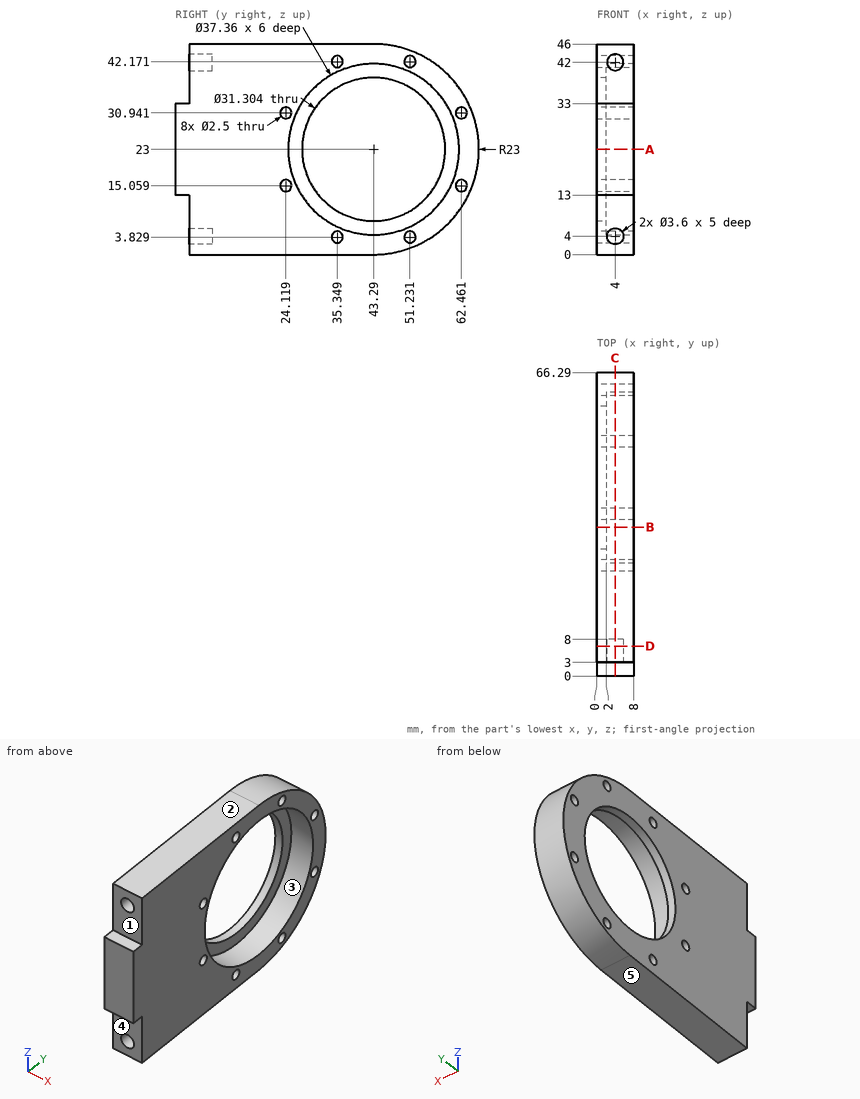
Verification items for this drawing (mm, ordinates from the low corner). A direction names the side the tool comes from. Give positions to 0.01 mm unless a question says otherwise; leave off trailing zeros. Write each loop counter-clockwise with the first axis right and the second up, starting at its lowest first coordinate (ties: lowest second). Pieces come first, ordered by that corner, then holes. Notation, with made-up numbers: M -37,62.25 L -9,62.25 A10 ccw -9,69.25 Z; hole C -33.5,-9.5 d6. An arc over 180 degrees is marked long. Use one line per item in the form item = value.
(1) Draft check along Z on the marked faces 3, 4 and 5. Enter one of: pulls with the +Z half, pulls with the -Z half, needs draft (parallel to the pull), parting line crosses it, or undercut.
Answer block:
face_3 = undercut
face_4 = needs draft
face_5 = pulls with the -Z half
(2) Tool access check on the marked faces 1 and 2. Record the directions out of +Z, -Z, +X, -X, +Y, -Y that give a thin tool (end or side, any length) a straight path to the whole face; none if there is none.
Answer block:
face_1 = +Z, +X, -X, -Y
face_2 = +Z, +X, -X, +Y, -Y
(3) Section check B-B on y = 32.5. Record the boundary of the cut face in (x, z).
Answer block:
outline = M 0,0 L 8,0 L 8,7.75 L 2,7.75 L 2,11.66 L 0,11.66 Z; M 0,34.34 L 2,34.34 L 2,38.25 L 8,38.25 L 8,46 L 0,46 Z
(4) Material ranges on line 1 along X through (y, z) = (6, 4); line 2 along Y through (x, z) = (1.25, 16) (1 decimal); line 3 along Y through (x, z) = (3.75, 30.5), recorded low to high.
Answer block:
line_1 = 0 to 2.2, 5.8 to 8
line_2 = 0 to 23.3, 24.9 to 29.3, 57.3 to 61.6, 63.3 to 65.2
line_3 = 0 to 22.95, 25.29 to 26.18, 60.4 to 61.29, 63.63 to 65.03
(5) Depth check by flat-ended pin: P1, Ø0.9, axis at x = 5, y = 2, coming from the -Z side; P2, Ø19, axis at y = 43.29, z = 23, coming from the -X side; P3, Ø1.8, axis at x = 3.5, z = 4.5, coming from the -Y side; P4, Ø3.5, axis at x = 4, y = 1, coming from the +Z side. Enter the tip coordinate at first touch or a pass-through.
Answer block:
P1 = 13
P2 = through
P3 = 8
P4 = 33
(6) Section check C-C on x = 4. State how many separate pieces and enclosed holes the cut face has, plus the area to 3 significant figures.
Answer block:
separate_pieces = 1
enclosed_holes = 9
area = 1,570 mm2
(7) Section check A-A on z = 23. Record the boundary of the cut face in (x, y).
Answer block:
outline = M 0,0 L 8,0 L 8,24.61 L 2,24.61 L 2,27.64 L 0,27.64 Z; M 0,58.94 L 2,58.94 L 2,61.97 L 8,61.97 L 8,66.29 L 0,66.29 Z
(8) Section check D-D on y = 6.5. Record the boundary of the cut face in (x, z), plus the area to 3 significant figures.
Answer block:
outline = M 0,0 L 8,0 L 8,46 L 0,46 Z; hole C 4,4 d3.6; hole C 4,42 d3.6
area = 348 mm2
